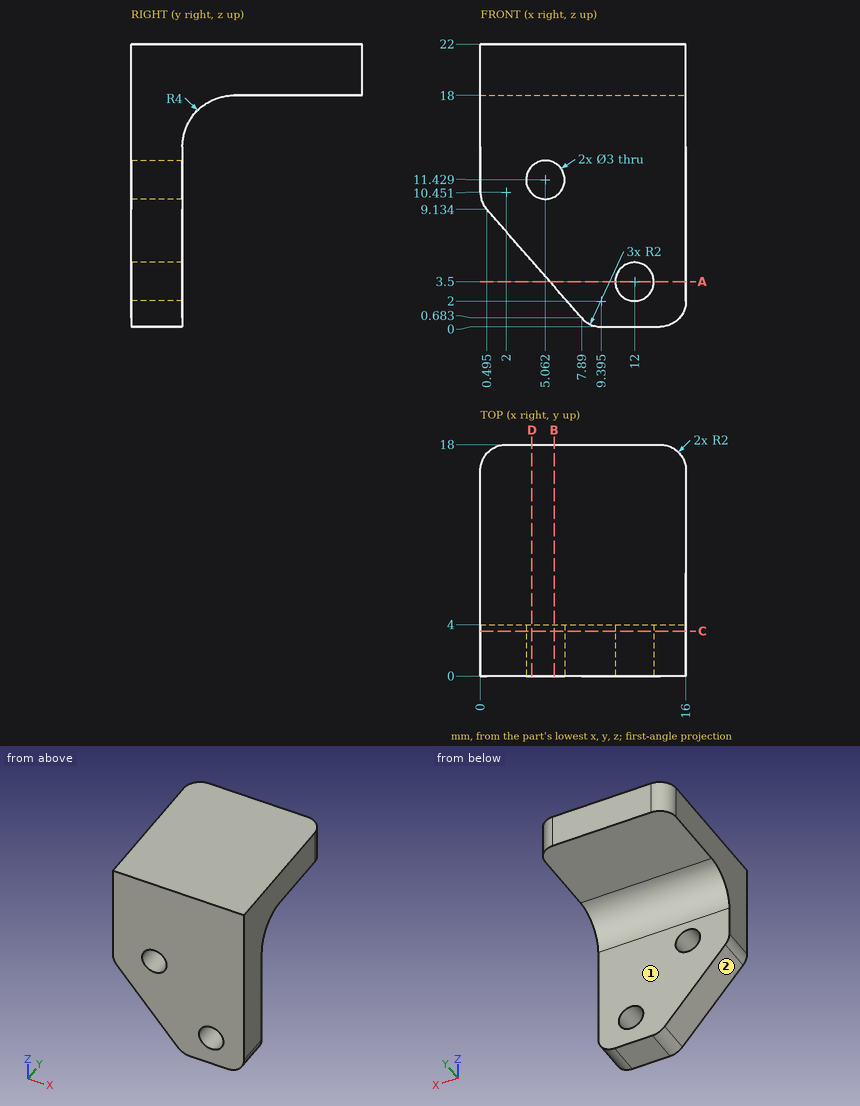
Drawing for the job (mm, zero at the part's lowest x, y, z). A direction names the side the tool comes from. Round coordinates to 2 decimals unless told otherwise and drop trailing zeros. Order: outer loops, then holes, each group sorted by start corner. A loop starts at its lowest first (then second) coordinate and runs counter-clockwise, first axis right, second up.
Item 1: Probe line 1 along Z through (x, y) = (12, 2.05); line 2 along Y through (x, z) = (13.75, 9); line 3 along Z through (x, y) = (3.75, 14.25). List the from-to ranges inside material, lowest first.
Item 2: Saw through at B-B on x = 5.75. Write the cut outline in (y, z).
Item 3: Saw through at C-C on y = 3.5. Write the cut outline in (x, z) (1 decimal).
Item 4: Pin check, flat tips, straight feed: pin 1 (1 mm diameter, centred on x = 7.5, y = 12.5, fed in from -Z); pin 2 (5 mm diameter, centred on x = 12, z = 3.5, fed in from +Y); pin 3 (2 mm diameter, centred on x = 2.5, y = 2.5, fed in from -Z). Stop position of each tip, or through.
Item 5: Tool access for the marked faces 1 and 2: list every direction of +Z, -Z, +X, -X, +Y, -Y with a clear straight run to the whole face (end or side of a thin tool).
Item 6: Saw through at A-A on z = 3.5. Write the cut outline in (x, y) (1 decimal).
Item 7: Saw through at D-D on x = 4. Write the cut outline in (y, z).
Reported:
1. line 1: z = 0 to 2, 5 to 22
1. line 2: y = 0 to 4
1. line 3: z = 18 to 22
2. outline: (0, 3.13) - (4, 3.13) - (4, 10.1) - (0, 10.1) - close; (0, 12.76) - (4, 12.76) - (4, 14) arc R4 cw to (8, 18) - (18, 18) - (18, 22) - (0, 22) - close
3. outline: (0, 10.5) arc R2 ccw to (0.5, 9.1) - (7.9, 0.7) arc R2 ccw to (9.4, 0) - (14, 0) arc R2 ccw to (16, 2) - (16, 22) - (0, 22) - close; hole circle Ø3 at (5.1, 11.4); hole circle Ø3 at (12, 3.5)
4. pin 1: stops at z = 18
4. pin 2: stops at y = 4
4. pin 3: stops at z = 5.7
5. face 1: -Z, +X, -X, +Y
5. face 2: -Z, -X, +Y, -Y
6. outline: (5.4, 0) - (10.5, 0) - (10.5, 4) - (5.4, 4) - close; (13.5, 0) - (16, 0) - (16, 4) - (13.5, 4) - close
7. outline: (0, 5.13) - (4, 5.13) - (4, 10.37) - (0, 10.37) - close; (0, 12.49) - (4, 12.49) - (4, 14) arc R4 cw to (8, 18) - (18, 18) - (18, 22) - (0, 22) - close
